For this review, take the finished solid that the model builds, in its own axes (mm). Round coordinates to 2 decimals unless told otherwise and drop trailing zeros. Use a Markdown table: item, result.
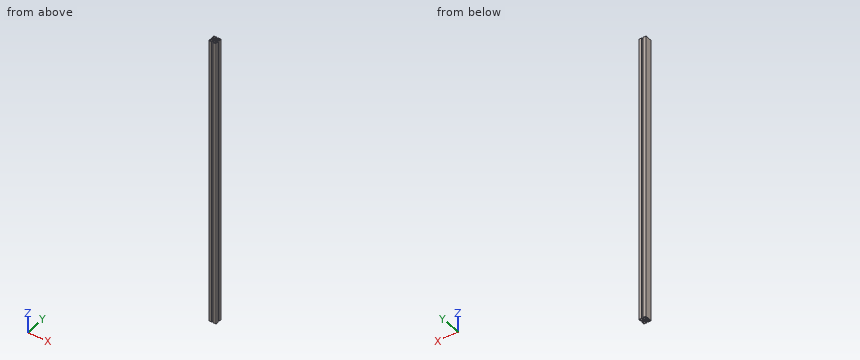
from build123d import *

# Parameters (mm, degrees)
SKETCH1_W           = 11.699975178
SKETCH1_H           = 11.699996949
SKETCH1_W_2         = 11.699990436
SKETCH1_H_2         = 11.699981689
SKETCH1_W_3         = 11.699990437
SKETCH1_H_3         = 11.699975177
SKETCH1_W_4         = 11.699981689
SKETCH1_H_4         = 11.699990436
BOSS_EXTRUDE1_DEPTH = 1816.1
CUT_EXTRUDE1_REACH  = 1818.1


with BuildPart() as part:
    # Sketch1 → Boss-Extrude1 (new body)
    with BuildSketch(Plane.XY):
        Polygon((22.500515052, 22.499297556), (-22.499484399, 22.499298105), (-22.499484948, -22.500701346), (-4.249491942, -22.500701568), (-4.249491942, -22.200733242), (-4.24949208, -18.000719999), (-6.799479919, -18.000719999), (-6.799480207, -9.200732353), (-4.799480391, -7.200732362), (4.800525817, -7.200732047), (6.8005258, -9.200731855), (6.800526088, -18.000720263), (4.250507877, -18.000720263), (4.250508015, -22.200733153), (4.250508015, -22.500701672), (22.500514502, -22.500701895), (22.500514725, -4.250714302), (22.200520351, -4.250714302), (18.000507108, -4.25071444), (18.000507108, -6.800702279), (9.200519462, -6.800702567), (7.200519471, -4.800702751), (7.200519156, 4.799303458), (9.200518964, 6.79930344), (18.000507424, 6.799303729), (18.000507424, 4.249285514), (22.200520261, 4.249285652), (22.500514829, 4.249285652), align=None)
        with BuildLine():
            Line((-4.249491247, 17.999291576), (-4.249490956, 22.199304807))
            Line((-4.249490956, 22.199304807), (-3.949472548, 22.199304807))
            Line((-3.949472548, 22.199304807), (-3.481695222, 21.73152644))
            ThreePointArc((-3.481695222, 21.73152644), (-2.670636178, 21.189593132), (-1.713926324, 20.999291428))
            Line((-1.713926324, 20.999291428), (1.714975167, 20.999291428))
            ThreePointArc((1.714975167, 20.999291428), (2.671722509, 21.189608628), (3.482801459, 21.731583767))
            Line((3.482801459, 21.731583767), (3.950490798, 22.199304487))
            Line((3.950490798, 22.199304487), (4.250509108, 22.199304487))
            Line((4.250509108, 22.199304487), (4.250508817, 17.999291575))
            Line((4.250508817, 17.999291575), (6.800527063, 17.999291575))
            Line((6.800527063, 17.999291575), (6.800526453, 9.199302988))
            Line((6.800526453, 9.199302988), (4.800526064, 7.199302969))
            Line((4.800526064, 7.199302969), (-4.799479817, 7.199303635))
            Line((-4.799479817, 7.199303635), (-6.799479854, 9.199304042))
            Line((-6.799479854, 9.199304042), (-6.799479244, 17.999291576))
            Line((-6.799479244, 17.999291576), (-4.249491247, 17.999291576))
        make_face(mode=Mode.SUBTRACT)
        with BuildLine():
            Line((-22.199510888, 4.249285566), (-17.999497356, 4.249285704))
            Line((-17.999497356, 4.249285704), (-17.999497356, 6.79927354))
            Line((-17.999497356, 6.79927354), (-9.199509947, 6.799273828))
            Line((-9.199509947, 6.799273828), (-7.199509956, 4.799274012))
            Line((-7.199509956, 4.799274012), (-7.199509641, -4.800732197))
            Line((-7.199509641, -4.800732197), (-9.199509449, -6.800732179))
            Line((-9.199509449, -6.800732179), (-17.99949762, -6.800732468))
            Line((-17.99949762, -6.800732468), (-17.99949762, -4.250714253))
            Line((-17.99949762, -4.250714253), (-22.199510799, -4.250714391))
            Line((-22.199510799, -4.250714391), (-22.199510799, -3.950696126))
            Line((-22.199510799, -3.950696126), (-21.731790056, -3.48300681))
            ThreePointArc((-21.731790056, -3.48300681), (-21.189814855, -2.671927844), (-20.999497617, -1.71518046))
            Line((-20.999497617, -1.71518046), (-20.999497617, 1.713721031))
            ThreePointArc((-20.999497617, 1.713721031), (-21.189799286, 2.670430863), (-21.731732544, 3.481489907))
            Line((-21.731732544, 3.481489907), (-22.199510888, 3.949267256))
            Line((-22.199510888, 3.949267256), (-22.199510888, 4.249285566))
        make_face(mode=Mode.SUBTRACT)
        with Locations((-14.649542346, -14.650709384)):
            Rectangle(SKETCH1_W, SKETCH1_H, mode=Mode.SUBTRACT)
        with Locations((14.65050626, -14.650767962)):
            Rectangle(SKETCH1_W_2, SKETCH1_H_2, mode=Mode.SUBTRACT)
        with BuildLine():
            Line((-3.181457266, -4.596908447), (-4.595670829, -3.182694885))
            Line((-4.595670829, -3.182694885), (-3.26221457, -1.849238626))
            ThreePointArc((-3.26221457, -1.849238626), (-3.749476751, -0.00071437), (-3.26221457, 1.847809887))
            Line((-3.26221457, 1.847809887), (-4.595670829, 3.181266146))
            Line((-4.595670829, 3.181266146), (-3.181457266, 4.595479708))
            Line((-3.181457266, 4.595479708), (-1.848001007, 3.262023449))
            ThreePointArc((-1.848001007, 3.262023449), (0.000523249, 3.74928563), (1.849047505, 3.262023449))
            Line((1.849047505, 3.262023449), (3.182503764, 4.595479708))
            Line((3.182503764, 4.595479708), (4.596717327, 3.181266146))
            Line((4.596717327, 3.181266146), (3.263261068, 1.847809887))
            ThreePointArc((3.263261068, 1.847809887), (3.750523249, -0.00071437), (3.263261068, -1.849238626))
            Line((3.263261068, -1.849238626), (4.596717327, -3.182694885))
            Line((4.596717327, -3.182694885), (3.182503764, -4.596908447))
            Line((3.182503764, -4.596908447), (1.849047505, -3.263452188))
            ThreePointArc((1.849047505, -3.263452188), (0.000523249, -3.75071437), (-1.848001007, -3.263452188))
            Line((-1.848001007, -3.263452188), (-3.181457266, -4.596908447))
        make_face(mode=Mode.SUBTRACT)
        with Locations((-14.64949028, 14.649335967)):
            Rectangle(SKETCH1_W_3, SKETCH1_H_3, mode=Mode.SUBTRACT)
        with Locations((14.650561583, 14.6492839)):
            Rectangle(SKETCH1_W_4, SKETCH1_H_4, mode=Mode.SUBTRACT)
    extrude(amount=BOSS_EXTRUDE1_DEPTH)

    # Sketch1_4 → Cut-Extrude1 (cut, up to next)
    with BuildSketch(Plane.XY, mode=Mode.PRIVATE) as cut_extrude1_sk1:
        with BuildLine():
            Line((-4.249490956, 22.499297883), (-4.249490956, 22.199304807))
            Line((-4.249490956, 22.199304807), (-3.949472548, 22.199304807))
            Line((-3.949472548, 22.199304807), (-3.481695222, 21.73152644))
            ThreePointArc((-3.481695222, 21.73152644), (-2.670636178, 21.189593132), (-1.713926324, 20.999291428))
            Line((-1.713926324, 20.999291428), (1.714975167, 20.999291428))
            ThreePointArc((1.714975167, 20.999291428), (2.671722509, 21.189608628), (3.482801459, 21.731583767))
            Line((3.482801459, 21.731583767), (3.950490798, 22.199304487))
            Line((3.950490798, 22.199304487), (4.250509108, 22.199304487))
            Line((4.250509108, 22.199304487), (4.250509108, 22.499297779))
            Line((4.250509108, 22.499297779), (-4.249490956, 22.499297883))
        make_face()
    cut_extrude1_tool1 = extrude(cut_extrude1_sk1.sketch, amount=CUT_EXTRUDE1_REACH, mode=Mode.PRIVATE) & part.part
    add(cut_extrude1_tool1.solids().sort_by_distance((0.000518, 21.824215, 0))[0], mode=Mode.SUBTRACT)


solid = part.part
Q1. Clearance check with a flat-ended pin moving along its axis: pin 1 (4 mm diameter, centred on x = 9.5, y = -15.5, fed in from -Z). State where the tip first meets the part, or that it passes through.
Determined:
| item | result |
|---|---|
| pin 1 | stops at z = 0 |
Q2. Wall thickness on line 1 along X through (y, z) = (0, 753); line 2 along Y through (x, z) = (10.5, 1242); line 3 along Y through (x, z) = (-4.5, 218): over which ranges is each line inside the solid? List them lowest first. Write a range as [from, to].
Determined:
| item | result |
|---|---|
| line 1 | x = [-22.5, -21], [-7.2, -3.75], [3.75, 7.2] |
| line 2 | y = [-22.5, -20.5], [-8.8, -6.8], [6.8, 8.8], [20.5, 22.5] |
| line 3 | y = [-22.5, -18], [-7.2, -3.28], [-3.09, 3.09], [3.28, 7.2], [18, 22.5] |
Q3. Add section A-A (z = 1518.5). Give the number of separate pieces and of enclosed holes in the cut face, then the cut area to 3 significant figures.
Determined:
| item | result |
|---|---|
| separate pieces | 1 |
| enclosed holes | 6 |
| area | 705 mm^2 |
